Geometry check sheet. Reference: the model listing, model coordinates, mm. Face numbers are marked on the shaded views. A direction names the side the tool comes from. Give positions to 0.01 mm unless a question says otherwise; leave off trailing zeros. Write each loop counter-clockwise with the first axis right and the second up, starting at its lowest first coordinate (ties: lowest second). Pieces come first, ordered by that corner, then holes.
(1) Depth check by flat-ended pin: P1, Ø2, axis at y = 2.5, z = 1.5, coming from the +X side; P2, Ø3, axis at x = -0.5, y = -0.5, coming from the -Z side; P3, Ø1, axis at y = 2.5, z = 4, coming from the +X side. Enter the tip coordinate at first touch or a pass-through.
(2) Thickness scan on line 1 along Y through (x, z) = (0, 2.5); line 2 along Y through (x, z) = (0, 4.7); line 3 along X through (y, z) = (0, 0.4). Record the ranges inside material, lowest first.
(3) Mould release check, pull along Y, two halves, no side actions. Record for the marked faces 4, 5 and 6: +Y half, -Y half, draft (parallel to the pull), parting line (faces both ways), or undercut.
(4) Cross-section at C-C (z = 4.6). Record the boundary of the cut face in (x, y).
(5) Tool access check on the marked faces 1, 2 and 3. Record the directions out of +Z, -Z, +X, -X, +Y, -Y that give a thin tool (end or side, any length) a straight path to the whole face; none if there is none.
```python
from build123d import *

# Parameters (mm, degrees)
F1_ANGLE_BACK = 135
F1_ANGLE      = 270
F2_SIZE       = 0.4
F3_SIZE       = 1.44999


# Not quite as in the source:
# - a fillet or chamfer is up to 0.001 mm smaller than in the source, because OpenCascade refuses the exact size


with BuildPart() as f1:
    # F0 (on Front) → F1 (revolve)
    with BuildSketch(Plane.XZ, mode=Mode.PRIVATE) as f1_sk:
        Polygon((2.65, 1.5), (2.65, 0), (4, 0), (4, 5), (2.15, 5), (2.15, 3), (3.6, 3), (3.6, 1.5), align=None)
    revolve(f1_sk.sketch.rotate(Axis((0, 0, 2.5), (0, 0, -1)), -F1_ANGLE_BACK), axis=Axis((0, 0, 2.5), (0, 0, -1)), revolution_arc=F1_ANGLE)

    # F2
    f2_edges = [f1.edges().sort_by_distance(p)[0] for p in [
        (2.65, 0, 1.5),
    ]]
    chamfer(f2_edges, length=F2_SIZE)

    # F3 (size 1.45 in the source; OpenCascade refuses exactly that, so slightly less here)
    f3_edges = [f1.edges().sort_by_distance(p)[0] for p in [
        (2.15, 0, 3),
    ]]
    chamfer(f3_edges, length=F3_SIZE)


solid = f1.part
```
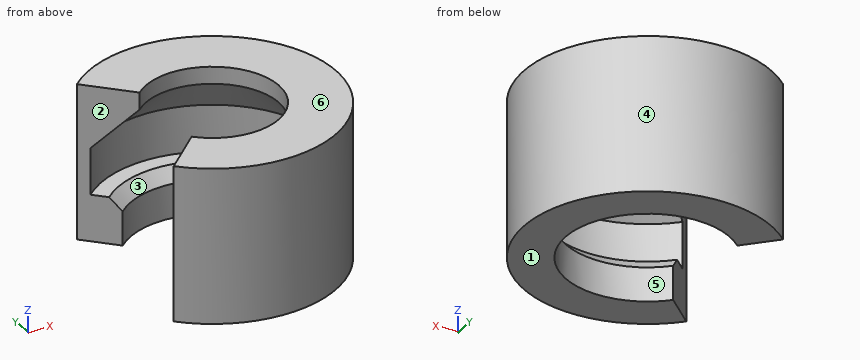
Reply:
1. P1: stops at x = 3.71
1. P2: stops at z = 4.39
1. P3: stops at x = 3.46
2. line 1: y = -4 to -3.6, 3.6 to 4
2. line 2: y = -4 to -2.15, 2.15 to 4
2. line 3: x = 2.65 to 4
3. face 4: parting line
3. face 5: undercut
3. face 6: draft
4. outline: (-2.83, -2.83) arc R4 ccw (long way) to (-2.83, 2.83) - (-1.52, 1.52) arc R2.15 cw (long way) to (-1.52, -1.52) - close
5. face 1: -Z, +X, -X, +Y, -Y
5. face 2: +Z, -Z, -X
5. face 3: none
